Could you check a few things on this model? Use its own coordinates, in mm. A direction names the side the tool comes from. Round coordinates to 2 decimals unless told otherwise and drop trailing zeros. Order: outer loops, then holes, each group sorted by start corner. A loop starts at its lowest first (then second) coordinate and runs counter-clockwise, first axis right, second up. Notation, with made-up numbers: (-7.75, -29.5) - (19.25, -29.5) arc R13 cw to (19.25, -25.5) - close; hole circle Ø10 at (13.5, 8.25). An arc over 180 degrees is marked (long way). Use one line per item in the form item = value.
from build123d import *

# Parameters (mm, degrees)
SKETCH_1_W               = 170
SKETCH_1_H               = 97
EXTRUDE_1_DEPTH          = 27
CUT_EXTRUDE_1_DEPTH      = 198.580363397
CUT_EXTRUDE_1_DEPTH_BACK = 198.580363397
SKETCH_4_W               = 2
SKETCH_4_H               = 2
CUT_EXTRUDE_2_DEPTH      = 198.580363397
SKETCH_5_R               = 18.5
SKETCH_5_R_2             = 2
CUT_EXTRUDE_3_DEPTH      = 197.959386677
SKETCH_6_R               = 3
CUT_EXTRUDE_4_DEPTH      = 2


with BuildPart() as part:
    # 草图1 → 凸台-拉伸1 (new body)
    with BuildSketch(Plane.XY):
        with Locations((-85, -48.5)):
            Rectangle(SKETCH_1_W, SKETCH_1_H)
    extrude(amount=EXTRUDE_1_DEPTH)

    # 草图2 → 切除-拉伸1 (cut, two sides: drawn at the far end of the back side and taken through both)
    with BuildSketch(Plane(origin=(0, 0, 0), x_dir=(1, 0, 0), z_dir=(0, 1, 0)).offset(-CUT_EXTRUDE_1_DEPTH_BACK)):
        Polygon((-5, -5), (-165, -5), (-165, -25), (-163, -25), (-163, -27), (-7, -27), (-7, -25), (-5, -25), align=None)
    extrude(amount=CUT_EXTRUDE_1_DEPTH + CUT_EXTRUDE_1_DEPTH_BACK, mode=Mode.SUBTRACT)

    # 草图4 → 切除-拉伸2 (cut, through all)
    with BuildSketch(Plane(origin=(0, 0, 0), x_dir=(1, 0, 0), z_dir=(0, 1, 0))):
        with Locations((-6, -26)):
            Rectangle(SKETCH_4_W, SKETCH_4_H)
        with Locations((-164, -26)):
            Rectangle(SKETCH_4_W, SKETCH_4_H)
    extrude(amount=-CUT_EXTRUDE_2_DEPTH, mode=Mode.SUBTRACT)

    # 草图5 → 切除-拉伸3 (cut, through all)
    with BuildSketch(Plane.XY.offset(5)):
        with Locations((-113, -48.5)):
            Circle(SKETCH_5_R)
        with Locations((-108, -12.7)):
            Circle(SKETCH_5_R_2)
        with Locations((-108, -84.3)):
            Circle(SKETCH_5_R_2)
        with Locations((-52, -12.7)):
            Circle(SKETCH_5_R_2)
        with Locations((-52, -84.3)):
            Circle(SKETCH_5_R_2)
    extrude(amount=-CUT_EXTRUDE_3_DEPTH, mode=Mode.SUBTRACT)

    # 草图6 → 切除-拉伸4 (cut)
    with BuildSketch(Plane.XY.offset(5)):
        with Locations((-108, -12.7)):
            Circle(SKETCH_6_R)
        with Locations((-52, -12.7)):
            Circle(SKETCH_6_R)
        with Locations((-108, -84.3)):
            Circle(SKETCH_6_R)
        with Locations((-52, -84.3)):
            Circle(SKETCH_6_R)
    extrude(amount=-CUT_EXTRUDE_4_DEPTH, mode=Mode.SUBTRACT)


solid = part.part
Item 1: Will these pins go through, and if not, where does the flat tip stop? P1, Ø1.8, axis at x = -109.5, y = -13, coming from the +Z side; P2, Ø1, axis at x = -90, y = -22, coming from the -Z side; P3, Ø8, axis at x = -52, y = -12.7, coming from the +Z side.
Found:
P1 = 3
P2 = 0
P3 = 5
Item 2: For faces 4 (the face through (-85, 0, 3)), 5 (the face through (-55, -12.6, 4)), 6 (the face through (-165, -49, 16)), which set-ups out of +Z, -Z, +X, -X, +Y, -Y let a thin tool reach every point of the face, with its end or its side?
Found:
face_4 = +Z, -Z, +X, -X, +Y
face_5 = +Z
face_6 = +Z, +Y, -Y
Item 3: Imagine slicing it at C-C on z = 21.25. Please give me the cut outline in (x, y).
Found:
outline = (-170, -97) - (-165, -97) - (-165, 0) - (-170, 0) - close; (-5, -97) - (0, -97) - (0, 0) - (-5, 0) - close
Item 4: Imagine slicing it at D-D on x = -113. Please give me the cut outline in (y, z).
Found:
outline = (-97, 0) - (-67, 0) - (-67, 5) - (-97, 5) - close; (-30, 0) - (0, 0) - (0, 5) - (-30, 5) - close
Item 5: If we mould it in two halves opening along X, with no side actions, what happens to faces 1 (the face through (-86, -48, 0)), 2 (the face through (0, -49, 13)), 3 (the face through (-52, -82, 3))? For each: released by +X, released by -X, zero draft, split by the parting line, or undercut.
Found:
face_1 = zero draft
face_2 = released by +X
face_3 = undercut
Item 6: Imagine slicing it at A-A on y = -48.5. Please give me the cut outline in (x, z), plus the area to 3 significant figures.
Found:
outline = (-170, 0) - (-131.5, 0) - (-131.5, 5) - (-165, 5) - (-165, 27) - (-170, 27) - close; (-94.5, 0) - (0, 0) - (0, 27) - (-5, 27) - (-5, 5) - (-94.5, 5) - close
area = 885 mm2
Item 7: I need wall thicknesses on L1, parallel to Y at x = -52, z = 3.45; L2, parallel to X at y = -6, z = 23; L3, parallel to Z at x = -86, y = -57. Which ranges of each line are inside material? Lowest first, please.
Found:
L1 = -97 to -87.3, -81.3 to -15.7, -9.7 to 0
L2 = -170 to -165, -5 to 0
L3 = 0 to 5
Item 8: Imagine slicing it at B-B on x = -52. Please give me the cut outline in (y, z).
Found:
outline = (-97, 0) - (-86.3, 0) - (-86.3, 3) - (-87.3, 3) - (-87.3, 5) - (-97, 5) - close; (-82.3, 0) - (-14.7, 0) - (-14.7, 3) - (-15.7, 3) - (-15.7, 5) - (-81.3, 5) - (-81.3, 3) - (-82.3, 3) - close; (-10.7, 0) - (0, 0) - (0, 5) - (-9.7, 5) - (-9.7, 3) - (-10.7, 3) - close
